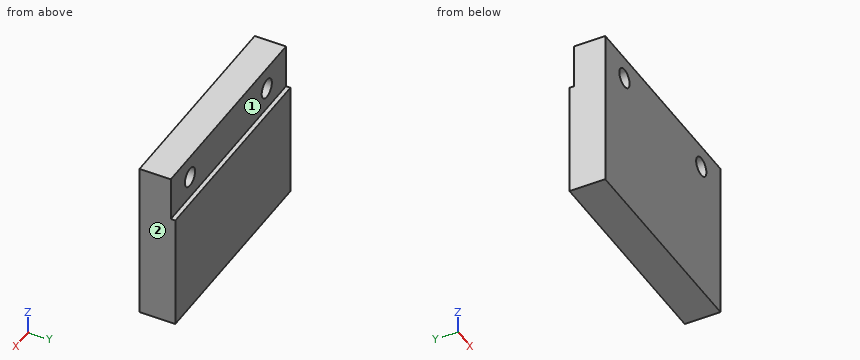
from build123d import *

# Parameters (mm, degrees)
F0_W     = 152.4
F0_H     = 114.3
F1_DEPTH = 25.4
F2_W     = 152.4
F2_H     = 31.75
F3_DEPTH = 3.175
F5_D     = 13.49248


with BuildPart() as f1:
    # F0 (on Front) → F1 (new body)
    with BuildSketch(Plane.XZ):
        Rectangle(F0_W, F0_H)
    extrude(amount=F1_DEPTH)

    # F2 (on face) → F3 (cut)
    with BuildSketch(Plane(origin=(0, 0, 0), x_dir=(-1, 0, 0), z_dir=(0, 1, 0))):
        with Locations((0, 41.275)):
            Rectangle(F2_W, F2_H)
    extrude(amount=-F3_DEPTH, mode=Mode.SUBTRACT)

    # F5 (through all)
    with Locations(Plane(origin=(0, -3.175, 0), x_dir=(-1, 0, 0), z_dir=(0, 1, 0))):
        with Locations((50.8, 41.275), (-50.8, 41.275)):
            Hole(F5_D / 2)


solid = f1.part
Check sheet for the modelled part. Datum: model origin and axes. Units: mm. Face numbers are marked on the shaded views. A direction names the side the tool comes from. Coordinates: 2 decimals unless noted, no trailing zeros. Write each loop counter-clockwise with the first axis right and the second up, starting at its lowest first coordinate (ties: lowest second). Pieces come first, ordered by that corner, then holes.
Item 1: Cross-section at A-A on x = -50.8. Record the boundary of the cut face in (y, z) (3 decimals).
Numbers:
outline: (-25.4, -57.15) - (0, -57.15) - (0, 25.4) - (-3.175, 25.4) - (-3.175, 34.529) - (-25.4, 34.529) - close; (-25.4, 48.021) - (-3.175, 48.021) - (-3.175, 57.15) - (-25.4, 57.15) - close
Item 2: Cross-section at C-C on x = 11. Record the boundary of the cut face in (y, z) (3 decimals).
Numbers:
outline: (-25.4, -57.15) - (0, -57.15) - (0, 25.4) - (-3.175, 25.4) - (-3.175, 57.15) - (-25.4, 57.15) - close
Item 3: Depth check by flat-ended pin: pin 1 Ø17.5 at (x, z) = (50.8, 41.275) entering from +Y (3 decimals); pin 2 Ø1.6 at (x, y) = (28, -2) entering from +Z. Enter the tip coordinate at first touch or a pass-through.
Numbers:
pin 1: stops at y = -3.175
pin 2: stops at z = 25.4
Item 4: Access from +Z, -Z, +X, -X, +Y, -Y to the whole of each face (thin tool, end or side, straight path). Record for the marked faces 1 and 2.
Numbers:
face 1: +Z, +X, -X, +Y
face 2: +Z, -Z, +X, +Y, -Y
Item 5: Cross-section at B-B on y = -10.25. Record the boundary of the cut face in (x, z) (3 decimals).
Numbers:
outline: (-76.2, -57.15) - (76.2, -57.15) - (76.2, 57.15) - (-76.2, 57.15) - close; hole circle Ø13.492 at (-50.8, 41.275); hole circle Ø13.492 at (50.8, 41.275)
Item 6: Scan lines: probe 1 along Z at (x, y) = (50.8, -14); probe 2 along Y at (x, z) = (17, 44) (3 decimals); probe 3 along Z at (x, y) = (7.5, -1.25). Record each from-to range of solid material in increasing order.
Numbers:
probe 1: z = -57.15 to 34.53, 48.02 to 57.15
probe 2: y = -25.4 to -3.175
probe 3: z = -57.15 to 25.4
